Autodesk Inventor part; units mm, degrees
ref_plane "YZ Plane" through (0, 0, 0) normal (1, 0, 0) x (0, 1, 0)
ref_plane "XZ Plane" through (0, 0, 0) normal (0, 1, 0) x (-1, 0, 0)
ref_plane "XY Plane" through (0, 0, 0) normal (0, 0, 1) x (1, 0, 0)
sketch "Sketch1" plane through (0, 0, 0) normal (0, 0, 1) x (1, 0, 0)
  line L0 (-12.5919, 2.2112) -> (69.9581, 2.2112)
  line L1 (69.9581, 2.2112) -> (69.9581, 8.9549)
  line L2 (69.9581, 8.9549) -> (65.8687, 5.3862)
  line L3 (65.8687, 5.3862) -> (-12.5919, 5.3862)
  line L4 (-12.5919, 5.3862) -> (-12.5919, 2.2112)
  dimension "d0" = 3.175
  dimension "d2" = 4.0894
  dimension "d3" = 6.7437
  dimension "d19" = 82.55
revolve "Revolution1" add sketch "Sketch1" angle 360 about axis through (-12.5919, 2.2112, 0) along (1, 0, 0)
thread "Thread1"
sketch "Sketch2" plane through (69.9581, 2.2112, 0) normal (1, 0, 0) x (0, 0, -1)
  circle A0 centre (0, 0) radius 6.7437
  line L0 (0, -2.2914) -> (-1.9844, -1.1457)
  line L1 (-1.9844, -1.1457) -> (-1.9844, 1.1457)
  line L2 (-1.9844, 1.1457) -> (0, 2.2914)
  line L3 (0, 2.2914) -> (1.9844, 1.1457)
  line L4 (1.9844, 1.1457) -> (1.9844, -1.1457)
  line L5 (1.9844, -1.1457) -> (0, -2.2914)
  dimension "d16" = 3.9688
extrude "Extrusion1" cut sketch "Sketch2" against normal blind 1.905 contours L0 L1 L2 L3 L4 L5
properties part number "HW-00073"
Can you work these out from the model? Positions are in its coordinate system, mm. A direction names the side the tool comes from. Give positions to 0.01 mm unless a question says otherwise; leave off trailing zeros. Loops run counter-clockwise (first coordinate to the right, second up) from the corner with the lowest first, then second, coordinate; pieces in that order, holes last. Notation, with made-up numbers: M -36,31.5 L -3,31.5 A17 cw -3,49.5 Z; hole C 45.25,-19.75 d3. An arc over 180 degrees is marked long. Use CSV: the item, a comma, the result in double quotes. Start each with the question number.
1. For P1, Ø3, axis at x = 33, y = 2.5, coming from the -Z side (3 decimals); P2, Ø3, axis at x = 18.5, y = 5.5, coming from the +Z side; P3, Ø8, axis at x = -1.5, y = 6, coming from the +Z side (3 decimals), each with a flat end and sliding along its axis, tell me the tip position at first contact or that it passes through.
2. If we mould it in two halves opening along Y, with no side actions, what happens to faces 1 (the face through (69.02, 3.92, 1.01)), 2 (the face through (69, 2, 1.984)), 3 (the face through (26.09, 5.24, -0.95)), 4 (the face through (69.958, 4, 2))? For each: released by +Y, released by -Y, zero draft, split by the parting line, or undercut.
3. On a 3-axis mill with a long thin cutter (end or side, diameter ignored), from which of +Z, -Z, +X, -X, +Y, -Y can I reach the whole of each face in a straight line? I mean faces 5 (the face through (69.019, 0.501, -1.006)), 6 (the face through (-12.592, 2, 0)). Say none if no direction works.
4. If I drill on L1, parallel to X at y = 3.75, z = 0.25; L2, parallel to X at y = 4, z = 3.5; L3, parallel to Y at x = -5.5, z = -0.75, over which ranges is the centre line in solid material (lowest first)?
5. Imagine slicing it at A-A, the plane x = 39.5. Write out the boundary of the cut face in (y, z) (3 decimals).
Response values:
1,P1,"z = -3.175"
1,P2,"z = 2.62"
1,P3,"z = 3.175"
2,face 1,"undercut"
2,face 2,"undercut"
2,face 3,"split by the parting line"
2,face 4,"zero draft"
3,face 5,"+X"
3,face 6,"+Z, -Z, -X, +Y, -Y"
4,L1,"-12.59 to 68.05"
4,L2,"66.73 to 69.96"
4,L3,"-0.87 to 5.3"
5,outline,"C 2.211,0 d6.35"
